Geometry: final body of the model. Coordinates: model frame, mm. A direction names the side the tool comes from. Coordinates: 2 decimals unless noted, no trailing zeros. Write each loop counter-clockwise with the first axis right and the second up, starting at its lowest first coordinate (ties: lowest second). Pieces come first, ordered by that corner, then holes. Notation, with made-up numbers: (16.25, -22.5) -> (44.25, -22.5) arc R27 cw to (44.25, 2.5) -> close; hole circle Ø4 at (-28, 45). An arc over 180 degrees is marked (long way). One line per item, written item: value. Start each with the question number.
Autodesk Inventor part; units mm, degrees
ref_plane "YZ Plane" through (0, 0, 0) normal (1, 0, 0) x (0, 1, 0)
ref_plane "XZ Plane" through (0, 0, 0) normal (0, 1, 0) x (-1, 0, 0)
ref_plane "XY Plane" through (0, 0, 0) normal (0, 0, 1) x (1, 0, 0)
sketch "Sketch1" plane through (0, 0, 0) normal (0, 0, 1) x (1, 0, 0)
  line L0 (-80, 0) -> (80, 0)
  line L1 (80, 0) -> (80, 50)
  line L2 (-80, 50) -> (-80, 0)
  line L3 (0, 116) -> (30, 116)
  line L4 (30, 116) -> (-30, 116)
  line L5 (-30, 116) -> (-80, 50)
  line L6 (30, 116) -> (80, 50)
  circle A0 centre (0, 92) radius 8
  circle A1 centre (0, 92) radius 12
  line L7 (80, 0) -> (80, -15)
  line L8 (80, -15) -> (55, -15)
  line L9 (55, -15) -> (55, 0)
  line L10 (-80, 0) -> (-80, -15)
  line L11 (-80, -15) -> (-55, -15)
  line L12 (-55, -15) -> (-55, 0)
  circle A2 centre (47, 25) radius 20
  circle A3 centre (-47, 25) radius 20
  circle A4 centre (0, 92) radius 20
  point P0 (0, 0)
  dimension "d0" = 160
  dimension "d1" = 50
  dimension "d3" = 60
  dimension "d4" = 16
  dimension "d5" = 24
  dimension "d6" = 15
  dimension "d7" = 25
  dimension "d12" = 40
  dimension "d13" = 40
  dimension "d21" = 40
extrude "Extrusion1" add sketch "Sketch1" along normal blind 20 contours L2 L5 L4 L3 L6 L1 L0 | L0 L12 L11 L10 | L0 L7 L8 L9 | A1 | A4
sketch "Sketch5" plane through (0, 0, 0) normal (0, 0, -1) x (-1, 0, 0)
  circle A0 centre (0, 92) radius 8
  circle A1 centre (0, 92) radius 20
  point P0 (0, 0)
  dimension "d22" = 40
extrude "Extrusion4" cut sketch "Sketch5" against normal blind 20
sketch "Sketch6" plane through (-55, 0, 0) normal (0, -1, 0) x (1, 0, 0)
  point P0 (55, 0)
sketch "Sketch7" plane through (-55, 0, 0) normal (0, -1, 0) x (1, 0, 0)
  line L0 (-25, 0) -> (-25, 20)
  line L1 (-12, 0) -> (28, 0)
  line L2 (-25, 20) -> (28, 20)
  line L3 (28, 20) -> (28, 0)
  line L4 (28, 0) -> (-25, 0)
  line L5 (-25, 0) -> (-25, 20)
  line L6 (135, 0) -> (135, 20)
  line L7 (135, 20) -> (82, 20)
  line L8 (82, 20) -> (82, 0)
  line L9 (82, 0) -> (135, 0)
  line L10 (135, 0) -> (135, 20)
  point P0 (55, 0)
  dimension "d25" = 53
extrude "Extrusion5" add sketch "Sketch7" along normal blind 45
sketch "Sketch8" plane through (-27, 0, 0) normal (0, -1, 0) x (1, 0, 0)
  line L0 (-40, 20) -> (0, 20)
  line L1 (57, 0) -> (-3, 0)
  line L2 (0, 20) -> (54, 20)
  line L3 (54, 20) -> (54, 0)
  line L4 (54, 0) -> (0, 0)
  line L5 (0, 0) -> (0, 20)
  point P0 (27, 0)
extrude "Extrusion6" add sketch "Sketch8" along normal blind 25
properties part number "Project_support_stand"
Q1. Cut plane B-B on z = 15.5. Output: boundary loops of the cut face in (x, y), and give its area (3 significant figures).
Q2. Cut plane D-D on y = 92. Output: boundary loops of the cut face in (x, z).
Q3. Access query for faces 5 (the flat face through (55, 83, 10)), 6 (the flat face through (-27, -35, 10)). Directions: +Z, -Z, +X, -X, +Y, -Y. A direction counts if a zero-diameter tool reaches every point of the face in a straight line with its end or side. Return the directions, or none.
Q4. Line query: L1, parallel to X at y = 26, z = 1; L2, parallel to Y at x = 0, z = 11; L3, parallel to X at y = 9.5, z = 18.25. Output: solid intervals per line, ascending. Write a range as from..to.
Q5. Cut plane C-C on y = 25. Output: boundary loops of the cut face in (x, z).
Q6. Cut plane A-A on x = 47. Output: boundary loops of the cut face in (y, z).
Q7. Draft query along Y for faces 1 (the flat face through (27, -35, 10)), 2 (the flat face through (-54, -45, 10)), 3 (the cylindrical face through (-28.525, 32.66, 9.86)), 4 (the cylindrical face through (4.336, 72.476, 9.86)). Return one class per face: pulls with the +Y half, pulls with the -Y half, needs draft (parallel to the pull), parting line crosses it, or undercut.
Q8. First-contact query: P1, Ø1, axis at x = 16, z = 3.5, coming from the -Y side; P2, Ø4, axis at y = 59.5, z = 13.5, coming from the +X side. Flat tips, straight axial feed; report the tip coordinate or a pass-through.
Solution:
1. outline: (-80, -45) -> (-27, -45) -> (-27, -25) -> (27, -25) -> (27, -45) -> (80, -45) -> (80, 50) -> (30, 116) -> (-30, 116) -> (-80, 50) -> close; hole circle Ø40 at (-47, 25); hole circle Ø40 at (0, 92); hole circle Ø40 at (47, 25)
1. area: 17,600 mm²
2. outline: (-48.18, 0) -> (-20, 0) -> (-20, 20) -> (-48.18, 20) -> close; (20, 0) -> (48.18, 0) -> (48.18, 20) -> (20, 20) -> close
3. face 5: +Z, -Z, +X, +Y
3. face 6: +Z, -Z, -Y
4. L1: -80..-66.97, -27.03..27.03, 66.97..80
4. L2: -25..72, 112..116
4. L3: -80..-59.64, -34.36..34.36, 59.64..80
5. outline: (-80, 0) -> (-67, 0) -> (-67, 20) -> (-80, 20) -> close; (-27, 0) -> (27, 0) -> (27, 20) -> (-27, 20) -> close; (67, 0) -> (80, 0) -> (80, 20) -> (67, 20) -> close
6. outline: (-45, 0) -> (5, 0) -> (5, 20) -> (-45, 20) -> close; (45, 0) -> (93.56, 0) -> (93.56, 20) -> (45, 20) -> close
7. face 1: needs draft
7. face 2: pulls with the -Y half
7. face 3: undercut
7. face 4: undercut
8. P1: y = -25
8. P2: x = 74.32
